Model file for the job. Use its own axes, mm. Face numbers are marked on the shaded views. A direction names the side the tool comes from. Round coordinates to 2 decimals unless told otherwise and drop trailing zeros. Order: outer loops, then holes, each group sorted by start corner. A loop starts at its lowest first (then second) coordinate and runs counter-clockwise, first axis right, second up. Notation, with made-up numbers: (89.5, -17.75) -> (125.5, -17.75) arc R27 cw to (125.5, 21.25) -> close; hole circle Ø6 at (89.5, 39.25). An arc over 180 degrees is marked (long way). Put each result on its own line as item: value. Start each with the question number.
Q1. 3-axis set-ups, long thin cutter, end or side, ignore diameter. For the marked faces 1, 2 and 3: which of +Z, -Z, +X, -X, +Y, -Y reach the whole face in a straight line?
Q2. Cut at D-D, the plane x = 2.5. State how many separate pieces and enclosed holes the cut face has, and give its area (3 significant figures).
Q3. Probe L1, parallel to Y at x = 8.5, z = 14.5; L2, parallel to Y at x = 8.25, z = -11.5; L3, parallel to Y at x = 1.25, z = -16. List the from-to ranges inside material, lowest first.
Q4. Cut at B-B, the plane y = 5. List the corners of the cut face in (x, z).
Q5. Cut at A-A, the plane z = 0. List the corners of the cut face in (x, y).
Q6. Cut at C-C, the plane z = -32.5. List the corners of the cut face in (x, y), and give its area (3 significant figures).
Q7. Flat gauge pins, fed straight in: P1, Ø2, axis at x = 8.5, y = -24.5, coming from the +Z side; P2, Ø3, axis at x = 7, y = 5, coming from the +Z side; P3, Ø2, axis at x = 2.5, z = 32.73, coming from the +Y side; P4, Ø3, axis at y = -30.91, z = 10.04, coming from the -X side. Where does each tip first touch, or does it go through?
Q8. Pull direction Y, two halves, no side cores. Call the marked faces 4, 5 and 6: released by +Y, released by -Y, zero draft, split by the parting line, or undercut.
Autodesk Inventor part; units mm, degrees
ref_plane "YZ Plane" through (0, 0, 0) normal (1, 0, 0) x (0, 1, 0)
ref_plane "XZ Plane" through (0, 0, 0) normal (0, 1, 0) x (-1, 0, 0)
ref_plane "XY Plane" through (0, 0, 0) normal (0, 0, 1) x (1, 0, 0)
sketch "Skizze1" plane through (0, 0, 0) normal (1, 0, 0) x (0, 1, 0)
  arc A0 (10, 38.7298) -> (10, -38.7298) centre (0, 0) ccw
  line L0 (10, 38.7298) -> (10, -12)
  line L1 (10, -38.7298) -> (10, -25)
  line L2 (10, -12) -> (0, -12)
  line L3 (0, -12) -> (0, -25)
  line L4 (0, -25) -> (10, -25)
  circle A1 centre (0, 32.5) radius 2
  circle A2 centre (-19.103, 26.2931) radius 2
  circle A3 centre (-30.9093, 10.0431) radius 2
  circle A4 centre (-30.9093, -10.0431) radius 2
  circle A5 centre (-19.103, -26.2931) radius 2
  circle A6 centre (0, -32.5) radius 2
  circle A7 centre (0, 0) radius 1.25
  line L5 (-7, 0) -> (-24.8022, 3.139)
  line L6 (-24.8022, 3.139) -> (-24.8022, -3.139)
  line L7 (-24.8022, -3.139) -> (-7, 0)
  line L8 (-54.5, 0) -> (47, 0) construction
  line L9 (-18.5163, -16.7972) -> (-5.7341, -4.015)
  line L10 (-5.7341, -4.015) -> (-22.1172, -11.6546)
  line L11 (-22.1172, -11.6546) -> (-18.5163, -16.7972)
  line L12 (-5.5331, -24.38) -> (-2.3941, -6.5778)
  line L13 (-2.3941, -6.5778) -> (-11.4325, -22.2328)
  line L14 (-11.4325, -22.2328) -> (-5.5331, -24.38)
  line L15 (-18.5163, 16.7972) -> (-5.7341, 4.015)
  line L16 (-5.7341, 4.015) -> (-22.1172, 11.6546)
  line L17 (-22.1172, 11.6546) -> (-18.5163, 16.7972)
  line L18 (-5.5331, 24.38) -> (-2.3941, 6.5778)
  line L19 (-2.3941, 6.5778) -> (-11.4325, 22.2328)
  line L20 (-11.4325, 22.2328) -> (-5.5331, 24.38)
  circle A8 centre (0, 0) radius 25 construction
  circle A9 centre (0, 0) radius 32.5 construction
  point P0 (-24.8022, 0)
  dimension "d50" = 65
  dimension "d0" = 80
  dimension "d3" = 10
  dimension "d4" = 10
  dimension "d5" = 10
  dimension "d7" = 0
  dimension "d8" = 4
  dimension "d11" = 180
  dimension "d13" = 2.5
  dimension "d19" = 20
  dimension "d22" = 0
  dimension "d23" = 7
  dimension "d26" = 70
  dimension "d49" = 50
  dimension "d51" = 12
extrude "Extrusion1" add sketch "Skizze1" along normal blind 10
fillet "Rundung1" radius 1 15 edges at (5, -5.5331, -24.38) (5, -11.4325, -22.2328) (5, -18.5163, -16.7972) (5, -22.1172, -11.6546) (5, -24.8022, -3.139) (5, -24.8022, 3.139) (5, -18.5163, 16.7972) (5, -22.1172, 11.6546) (5, -11.4325, 22.2328) (5, -5.5331, 24.38) (5, -2.3941, 6.5778) (5, -5.7341, 4.015) (5, -7, 0) (5, -5.7341, -4.015) (5, -2.3941, -6.5778)
fillet "Rundung2" radius 2 4 edges at (5, 10, -12) (5, 0, -12) (5, 0, -25) (5, 10, -25)
sketch "Skizze2" plane through (10, 0, 0) normal (1, 0, 0) x (0, 0, -1)
  circle A0 centre (-16, 0) radius 0.75
  point P0 (0, 0)
  dimension "d30" = 1.5
  dimension "d31" = 16
extrude "Extrusion2" cut sketch "Skizze2" against normal blind 10
sketch "Skizze3" plane through (0, 2, -25) normal (0, 0, 1) x (1, 0, 0)
  circle A0 centre (7.5, 3) radius 1.25
  line L0 (10, 6) -> (10, 0)
  line L1 (0, 6) -> (10, 6)
  point P0 (0, -2)
  point P1 (10, 0.8802)
  dimension "d35" = 2.5
  dimension "d36" = 2.5
  dimension "d37" = 3
extrude "Extrusion3" cut sketch "Skizze3" against normal blind 12
sketch "Skizze4" plane through (0, 10, 38.7298) normal (0, 1, 0) x (1, 0, 0)
  circle A0 centre (2.5, 6) radius 1.25
  line L0 (0, 48.7298) -> (0, 0)
  line L1 (0, 0) -> (10, 0)
  point P0 (0, 38.7298)
  dimension "d40" = 2.5
  dimension "d41" = 2.5
  dimension "d42" = 6
extrude "Extrusion4" cut sketch "Skizze4" against normal blind 10
sketch "Skizze5" plane through (10, 0, 0) normal (1, 0, 0) x (0, 0, -1)
  circle A0 centre (0, 0) radius 1.25
  arc A1 (2.6458, -3) -> (-2.6458, -3) centre (0, 0) ccw
  line L0 (-2.6458, -3) -> (2.6458, -3)
  circle A2 centre (0, 0) radius 4
  line L1 (-2.6458, 3) -> (2.6458, 3)
  line L2 (0, 0) -> (0, 3) construction
  point P0 (-2.6458, -3)
  dimension "CapstonV2_ShaftDia" = 8
  dimension "Poligonprofil_Ausnehmung" = 1
  dimension "d52" = 1
extrude "Extrusion5" cut sketch "Skizze5" against normal blind 10 contours L0 A1 L1 | A2 L0
equation "\"d50\" = 0.5 * d0 + 0.5 * d49"
properties part number "Capstondisc_v2"
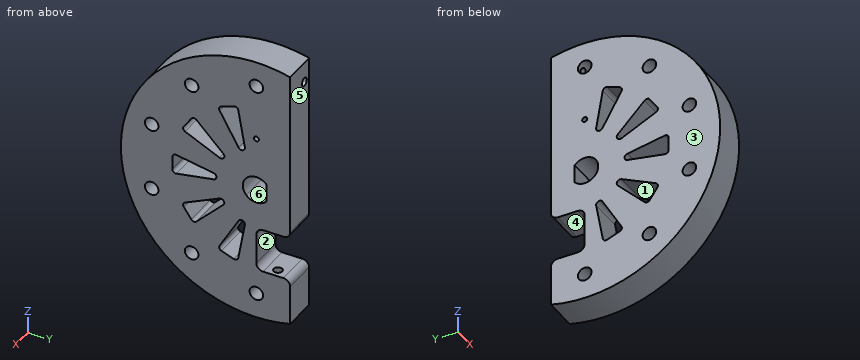
Ans:
1. face 1: +X, -X
1. face 2: +X, -X, +Y
1. face 3: +Z, -Z, -X, +Y, -Y
2. separate pieces: 1
2. enclosed holes: 12
2. area: 2,780 mm^2
3. L1: y = -37.28 to -20.12, -16.22 to -6.97, -3.79 to 10
3. L2: y = -38.31 to -32.28, -29.54 to -21.44, -13.22 to -5.24, -3.49 to 9.32
3. L3: y = -36.66 to -19.04, -17.72 to -7.83, -4.06 to 0
4. outline: (0, -39.69) -> (10, -39.69) -> (10, -25) -> (8.75, -25) -> (8.75, -37) -> (6.25, -37) -> (6.25, -25) -> (0, -25) -> close; (0, -12) -> (10, -12) -> (10, 39.69) -> (0, 39.69) -> close; hole circle Ø2.5 at (2.5, 32.73)
5. outline: (0, -40) -> (10, -40) -> (10, -24.8) -> (0, -24.8) -> close; (0, -11.76) -> (10, -11.76) -> (10, -4) -> (0, -4) -> close; (0, 3) -> (10, 3) -> (10, 10) -> (0, 10) -> close
6. outline: (0, -23.32) -> (10, -23.32) -> (10, -2) -> (0, -2) -> close; (0, 2) -> (10, 2) -> (10, 10) -> (0, 10) -> close; hole circle Ø2.5 at (7.5, 5)
6. area: 288 mm^2
7. P1: stops at z = 32.37
7. P2: stops at z = 39.85
7. P3: stops at y = -1.58
7. P4: passes through
8. face 4: zero draft
8. face 5: released by +Y
8. face 6: undercut
